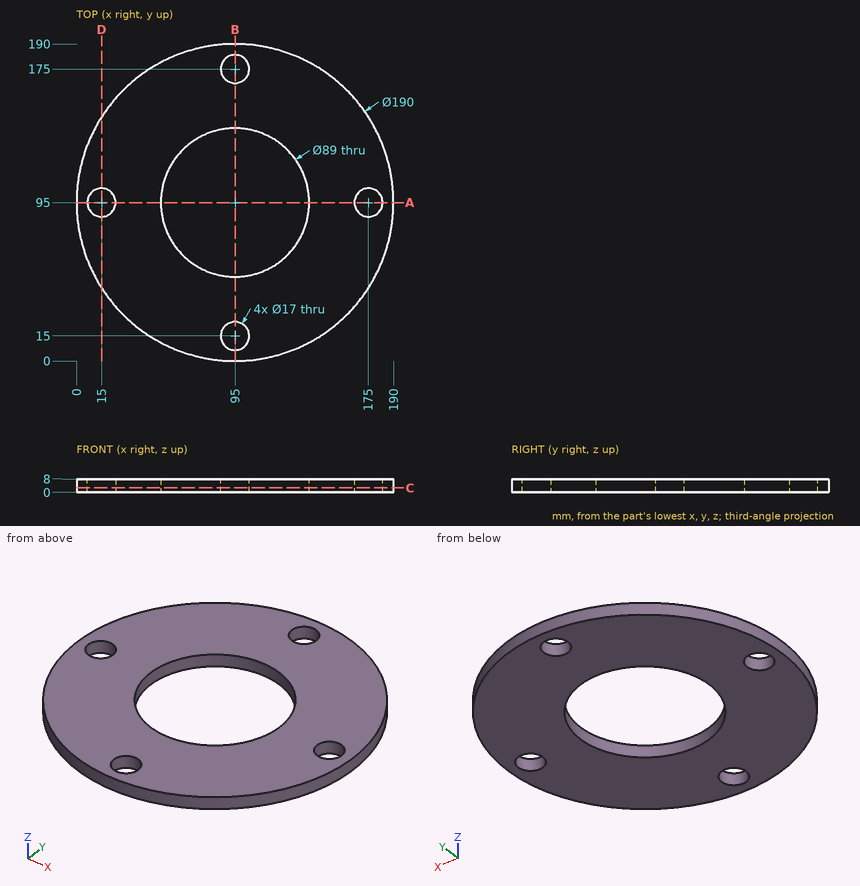
The drawing under review shows one solid part. Ordinate dimensions are in mm from its lowest x, y, z. Give positions to 0.01 mm unless a question says otherwise; leave off trailing zeros. Loops run counter-clockwise (first coordinate to the right, second up) from the corner with the lowest first, then second, coordinate; pieces in that order, holes last. Notation, with made-up numbers: M 30,-13 L 66,-13 A29 ccw 66,9 Z; hole C 55,71 d1. An arc over 180 degrees is marked long. Return JSON: item names as keys, results as strings. Group by question number.
Item 1: We need section D-D (x = 15). Give the boundary of the cut face in (y, z), and give its area (3 significant figures).
Item 2: Insertion check: pin 1 Ø1 at (x, z) = (41, 6) entering from -Y; pin 2 Ø4 at (y, z) = (30.5, 4) entering from -X; pin 3 Ø2 at (x, z) = (101, 1.5) entering from -Y. Each pin has a flat end and moves straight along its axis. Give the tip position at first contact, or say it passes through.
Item 3: We need section A-A (y = 95). Give the boundary of the cut face in (x, z).
Item 4: We need section C-C (z = 2.75). Give the boundary of the cut face in (x, y), and give its area (3 significant figures).
Item 5: For probe 1 along Y at (x, z) = (82, 6.5); probe 2 along Y at (x, z) = (178.5, 2.25); probe 3 along X at (y, z) = (132, 6), list the stretches that pass through material, from the lowest coordinate up.
Output:
{
 "1": {"outline": "M 43.77,0 L 86.5,0 L 86.5,8 L 43.77,8 Z; M 103.5,0 L 146.23,0 L 146.23,8 L 103.5,8 Z", "area": "684 mm^2"},
 "2": {"pin 1": "stops at y = 16.5", "pin 2": "stops at x = 23.45", "pin 3": "stops at y = 0.13"},
 "3": {"outline": "M 0,0 L 6.5,0 L 6.5,8 L 0,8 Z; M 23.5,0 L 50.5,0 L 50.5,8 L 23.5,8 Z; M 139.5,0 L 166.5,0 L 166.5,8 L 139.5,8 Z; M 183.5,0 L 190,0 L 190,8 L 183.5,8 Z"},
 "4": {"outline": "C 95,95 d190; hole C 15,95 d17; hole C 95,95 d89; hole C 95,15 d17; hole C 95,175 d17; hole C 175,95 d17", "area": "21,200 mm^2"},
 "5": {"probe 1": "y = 0.89 to 52.44, 137.56 to 189.11", "probe 2": "y = 49.69 to 87.25, 102.75 to 140.31", "probe 3": "x = 7.5 to 70.28, 119.72 to 182.5"}
}
